Build history of the part. All positions in model axes, mm. Face numbers are marked on the shaded views. A direction names the side the tool comes from. Coordinates: 2 decimals unless noted, no trailing zeros. Order: outer loops, then holes, each group sorted by start corner. A loop starts at its lowest first (then second) coordinate and runs counter-clockwise, first axis right, second up. Notation, with made-up numbers: (-25, -37.75) - (5, -37.75) arc R14 ccw to (5, -15.75) - close; hole circle Ø11 at (54.25, 58). An arc over 180 degrees is marked (long way). One line per item, written item: value.
from build123d import *

# Parameters (mm, degrees)
F0_W     = 14
F0_H     = 14
F1_DEPTH = 8.1
F2_W     = 18
F2_H     = 7.1
F3_DEPTH = 11.5
F5_DEPTH = 14
F6_W     = 11
F6_H     = 7.1
F7_DEPTH = 25


with BuildPart() as f1:
    # F0 (on Top) → F1 (new body)
    with BuildSketch(Plane.XY):
        Polygon((0, 11.5), (0, 0), (29.1, 0), (29.1, 11.5), (15.1, 11.5), align=None)
        with Locations((22.1, 18.5)):
            Rectangle(F0_W, F0_H)
    extrude(amount=F1_DEPTH)

    # F2 (on face) → F3 (cut)
    with BuildSketch(Plane.XZ):
        with Locations((20.1, 4.05)):
            Rectangle(F2_W, F2_H)
    extrude(amount=-F3_DEPTH, mode=Mode.SUBTRACT)

    # F4 (on face) → F5 (cut)
    with BuildSketch(Plane(origin=(0, 25.5, 0), x_dir=(-1, 0, 0), z_dir=(0, 1, 0))):
        with BuildLine():
            ThreePointArc((-17.741101, 0), (-16.562042, 1.874333), (-16.15, 4.05))
            ThreePointArc((-16.15, 4.05), (-16.562042, 6.225667), (-17.741101, 8.1))
            Line((-17.741101, 8.1), (-26.458899, 8.1))
            ThreePointArc((-26.458899, 8.1), (-28.05, 4.05), (-26.458899, 0))
            Line((-26.458899, 0), (-17.741101, 0))
        make_face()
    extrude(amount=-F5_DEPTH, mode=Mode.SUBTRACT)

    # F6 (on face) → F7 (cut)
    with BuildSketch(Plane(origin=(0, 0, 0), x_dir=(0, -1, 0), z_dir=(-1, 0, 0))):
        with Locations((-6, 4.05)):
            Rectangle(F6_W, F6_H)
    extrude(amount=-F7_DEPTH, mode=Mode.SUBTRACT)


solid = f1.part
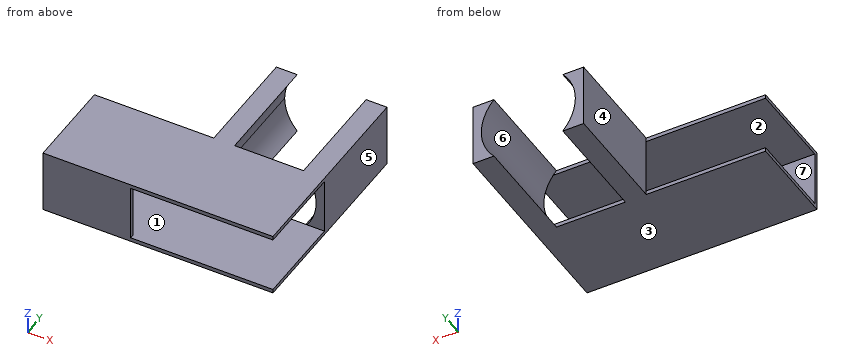
1. Probe line 1 along X through (y, z) = (19.5, 0.5); line 2 along Z through (x, y) = (19.75, 3.5); line 3 along Y through (x, z) = (10.25, 2.5). List the from-to ranges inside material, lowest first.
Values found:
line 1: x = 15.1 to 17.33, 26.87 to 29.1
line 2: z = 0 to 0.5, 7.6 to 8.1
line 3: y = 0 to 0.5
2. Band-saw the part on B-B, the plane x = 21.5. Give the cut face in (y, z).
Values found:
outline: (0, 0) - (11.5, 0) - (11.5, 0.5) - (0, 0.5) - close; (0, 7.6) - (11.5, 7.6) - (11.5, 8.1) - (0, 8.1) - close
3. Two-plate mould, pull along Z, no slides. Class the marked faces 1, 2, 3 and 4: pulls with the +Z half, pulls with the -Z half, needs draft (parallel to the pull), parting line crosses it, or undercut.
Values found:
face 1: undercut
face 2: undercut
face 3: pulls with the -Z half
face 4: needs draft
4. Band-saw the part on A-A, the plane y = 15. Give the cut face in (x, z).
Values found:
outline: (15.1, 0) - (17.74, 0) arc R5.95 cw to (16.15, 4.05) arc R5.95 cw to (17.74, 8.1) - (15.1, 8.1) - close; (26.46, 0) - (29.1, 0) - (29.1, 8.1) - (26.46, 8.1) arc R5.95 cw to start
5. Flat gauge pins, fed straight in: P1, Ø1.1, axis at x = 15.5, z = 4, coming from the -Y side; P2, Ø2, axis at x = 17.5, z = 4, coming from the -Y side; P3, Ø6, axis at x = 6.5, y = 9.5, coming from the -Z side; P4, Ø0.6, axis at x = 4.5, z = 8, coming from the +Y side. Where does each tip first touch, or does it go through?
Values found:
P1: stops at y = 11.5
P2: passes through
P3: stops at z = 0
P4: stops at y = 11.5
6. Band-saw the part on D-D, the plane y = 7.75. Give the cut face in (x, z).
Values found:
outline: (0, 0) - (29.1, 0) - (29.1, 0.5) - (0, 0.5) - close; (0, 7.6) - (29.1, 7.6) - (29.1, 8.1) - (0, 8.1) - close
7. Band-saw the part on C-C, the plane z = 5.5. Give the cut face in (x, y), and give its area (3 significant figures).
Values found:
outline: (0, 0) - (11.1, 0) - (11.1, 0.5) - (0, 0.5) - close; (15.1, 11.5) - (16.33, 11.5) - (16.33, 25.5) - (15.1, 25.5) - close; (27.87, 11.5) - (29.1, 11.5) - (29.1, 25.5) - (27.87, 25.5) - close
area: 40.0 mm2
8. 3-axis set-ups, long thin cutter, end or side, ignore diameter. For the marked faces 5, 6 and 7: which of +Z, -Z, +X, -X, +Y, -Y reach the whole face in a straight line?
Values found:
face 5: +Z, -Z, +X, +Y, -Y
face 6: +Y
face 7: +X, -X, +Y
